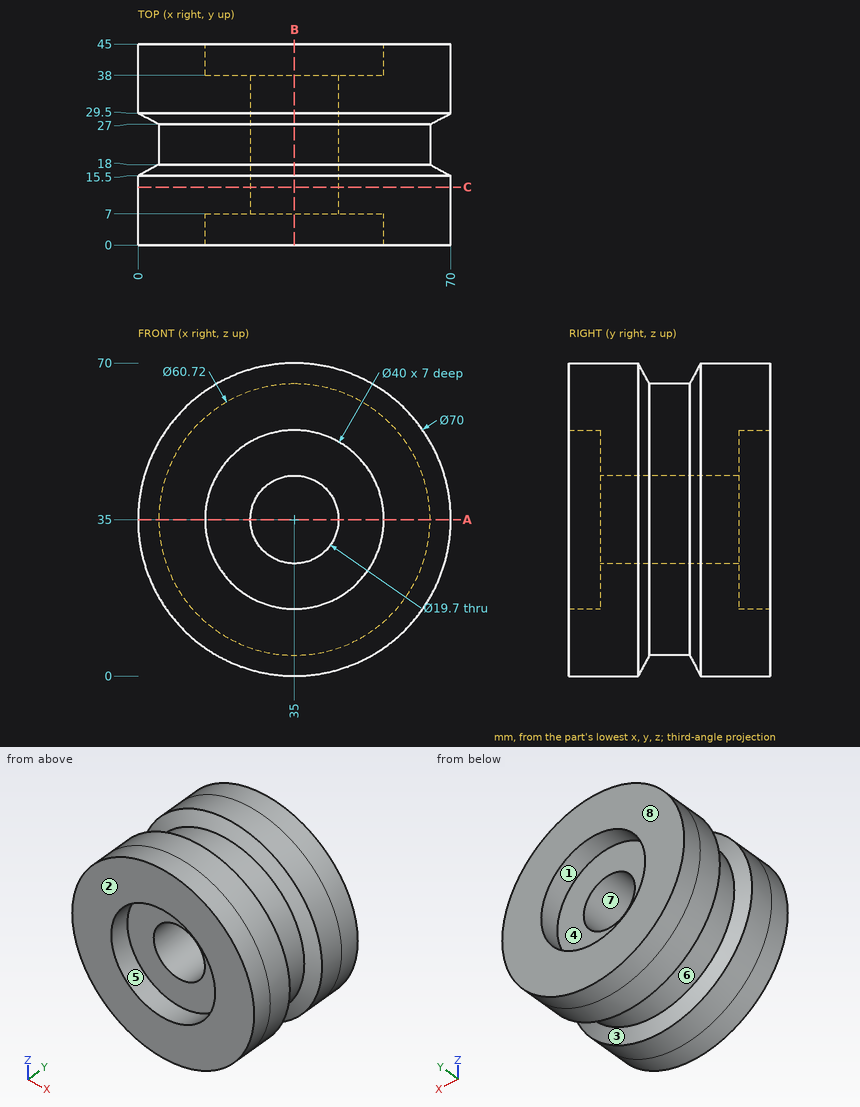
For this review, use the dimensioned drawing (mm, ordinates from the lowest corner) and the shaded views. A direction names the side the tool comes from. Round coordinates to 2 decimals unless told otherwise and drop trailing zeros. Write each loop counter-clockwise with the first axis right and the second up, starting at its lowest first coordinate (ties: lowest second). Pieces come first, ordered by that corner, then holes. Notation, with made-up numbers: (-20.5, 31.25) -> (21.5, 31.25) arc R23 cw to (21.5, 51.25) -> close; hole circle Ø4 at (8, 67.5). An arc over 180 degrees is marked (long way). Use one line per item in the form item = value.
Q1. Consider section C-C (y = 13). State the section outline as (x, z) points, then the cut area to 3 significant figures.
Resolved:
outline = circle Ø70 at (35, 35); hole circle Ø19.7 at (35, 35)
area = 3,540 mm²
Q2. To check wall thickness, follow probe 1 along X at (y, z) = (3.5, 35); probe 2 along Y at (x, z) = (46.5, 40); probe 3 along X at (y, z) = (6, 22). State the ranges of each line that lie inside material, in increasing order. Write a range as from..to.
Resolved:
probe_1 = 0..15, 55..70
probe_2 = 7..38
probe_3 = 2.5..19.8, 50.2..67.5
Q3. Clearance check with flat-ended pins moving along their axes: pin 1 Ø10 at (x, y) = (37.5, 29) entering from -Z; pin 2 Ø4 at (x, y) = (60.5, 28.5) entering from +Z; pin 3 Ø1 at (x, y) = (43, 8) entering from +Z; pin 4 Ø20 at (x, z) = (28, 31.5) entering from -Y. State where each tip first meets the part, or that it passes through.
Resolved:
pin_1 = 0
pin_2 = 60.69
pin_3 = 69.19
pin_4 = 7
Q4. Consider section A-A (z = 35). State the section outline as (x, y) points.
Resolved:
outline = (0, 0) -> (15, 0) -> (15, 7) -> (25.15, 7) -> (25.15, 38) -> (15, 38) -> (15, 45) -> (0, 45) -> (0, 29.5) -> (4.64, 27) -> (4.64, 18) -> (0, 15.5) -> close; (44.85, 7) -> (55, 7) -> (55, 0) -> (70, 0) -> (70, 15.5) -> (65.36, 18) -> (65.36, 27) -> (70, 29.5) -> (70, 45) -> (55, 45) -> (55, 38) -> (44.85, 38) -> close
Q5. Consider section B-B (x = 35). State the section outline as (y, z) points, then the cut area to 3 significant figures.
Resolved:
outline = (0, 0) -> (15.5, 0) -> (18, 4.64) -> (27, 4.64) -> (29.5, 0) -> (45, 0) -> (45, 15) -> (38, 15) -> (38, 25.15) -> (7, 25.15) -> (7, 15) -> (0, 15) -> close; (0, 55) -> (7, 55) -> (7, 44.85) -> (38, 44.85) -> (38, 55) -> (45, 55) -> (45, 70) -> (29.5, 70) -> (27, 65.36) -> (18, 65.36) -> (15.5, 70) -> (0, 70) -> close
area = 1,870 mm²
Q6. Machinability: for the marked faces 4, 5, 6, 7 and 8, which of the approach directions +Z, -Z, +X, -X, +Y, -Y give a long, thin tool a straight path to every point of the face, cutting with its end or side? Answer none if there is none.
Resolved:
face_4 = +Y
face_5 = -Y
face_6 = none
face_7 = +Y, -Y
face_8 = +Z, -Z, +X, -X, +Y
Q7. The part is to be moulded in two halves that separate along Y. For the marked faces 1, 2 and 3, say which applies: released by +Y, released by -Y, zero draft, split by the parting line, or undercut.
Resolved:
face_1 = zero draft
face_2 = released by -Y
face_3 = undercut
